```python
from build123d import *

# Parameters (mm, degrees)
F1_DEPTH = 12.7


with BuildPart() as f1:
    # F0 (on Front) → F1 (new body)
    with BuildSketch(Plane.XZ):
        Polygon((71.700338, 16.308149), (63.5, 12.7), (63.5, -12.7), (71.700338, -15.811923), align=None)
        with BuildLine():
            Line((63.5, 12.7), (-57.15, 12.7))
            ThreePointArc((-57.15, 12.7), (-61.640128, 10.840128), (-63.5, 6.35))
            Line((-63.5, 6.35), (-63.5, -6.35))
            ThreePointArc((-63.5, -6.35), (-61.640128, -10.840128), (-57.15, -12.7))
            Line((-57.15, -12.7), (63.5, -12.7))
            Line((63.5, -12.7), (63.5, 12.7))
        make_face()
    extrude(amount=F1_DEPTH)


solid = f1.part
```
Input: part model. Units: mm. Frame: model coordinates. A direction names the side the tool comes from. Give positions to 0.01 mm unless a question says otherwise; leave off trailing zeros. Order: outer loops, then holes, each group sorted by start corner. A loop starts at its lowest first (then second) coordinate and runs counter-clockwise, first axis right, second up. Notation, with made-up numbers: M 15.25,48 L 57.25,48 A23 ccw 57.25,74 Z; hole C 21,-35 d5. An arc over 180 degrees is marked long. Return JSON: item names as keys, results as strings.
Item 1: Cut plane A-A (y = -8.25). Return loops of the section in (x, z).
Solutions:
{"outline": "M -63.5,-6.35 A6.35 ccw -57.15,-12.7 L 63.5,-12.7 L 71.7,-15.81 L 71.7,16.31 L 63.5,12.7 L -57.15,12.7 A6.35 ccw -63.5,6.35 Z"}
Item 2: Cut plane B-B (x = 47). Return loops of the section in (y, z).
Solutions:
{"outline": "M -12.7,-12.7 L 0,-12.7 L 0,12.7 L -12.7,12.7 Z"}
Item 3: First-contact query: P1, Ø6, axis at x = -35, y = -1.5, coming from the +Z side; P2, Ø4, axis at y = -2.5, z = 10, coming from the -X side; P3, Ø6, axis at y = -2, z = -9, coming from the -X side; P4, Ø6.5, axis at x = 19.5, y = -4, coming from the -Z side. Flat tips, straight axial feed; report the tip coordinate or a pass-through.
Solutions:
{"P1": "z = 12.7", "P2": "x = -63.28", "P3": "x = -63.5", "P4": "z = -12.7"}
Item 4: Access query for faces 1 (the flat face through (2, -6, -12.7)), 2 (the flat face through (-63.5, -6, 0)), 3 (the flat face through (4, -6, 12.7)). Directions: +Z, -Z, +X, -X, +Y, -Y. A direction counts if a zero-diameter tool reaches every point of the face in a straight line with its end or side. Return the directions, or none.
Solutions:
{"face 1": "-Z, -X, +Y, -Y", "face 2": "+Z, -Z, -X, +Y, -Y", "face 3": "+Z, -X, +Y, -Y"}
Item 5: Ray query, probe 1 along Z at (x, y) = (-19, -9); probe 2 along X at (y, z) = (-6, 11.5); probe 3 along X at (y, z) = (-6, 15.5). Return the intervals inside material, ascending.
Solutions:
{"probe 1": "-12.7 to 12.7", "probe 2": "-60.86 to 71.7", "probe 3": "69.86 to 71.7"}
